For this review, take the finished solid that the model builds, in its own axes (mm). Round coordinates to 2 decimals unless told otherwise and drop trailing zeros. Order: outer loops, then holes, each group sorted by start corner. A loop starts at its lowest first (then second) coordinate and runs counter-clockwise, first axis right, second up. Notation, with made-up numbers: (-20, 31.25) - (35, 31.25) arc R15 ccw to (35, 56.25) - close; hole circle Ø3 at (0.5, 62). An arc over 180 degrees is marked (long way). Write each question's results on one line, items separated by ' | '. Start each with the question number.
(1) Take a section at C-C, the plane x = -2. Give the boundary of the cut face in (y, z).
(2) Take a section at D-D, the plane x = -51. Give the boundary of the cut face in (y, z).
(3) Take a section at A-A, the plane z = -15. Give the boundary of the cut face in (x, y), plus the area to 3 significant figures.
(4) For L1, parallel to Z at x = -38, y = 0.25; L2, parallel to Z at x = 28, y = 2.1; L3, parallel to Z at x = 12, y = 0.9, list the stretches that pass through material, from the lowest coordinate up. Write a range as from..to.
(5) Take a section at B-B, the plane y = 1.2. Give the boundary of the cut face in (x, z), plus the area to 3 significant figures.
(6) Insertion check: pin 1 Ø3 at (x, z) = (21.5, -17.5) entering from -Y. The pin has a flat end and moves straight along its axis. Give the tip position at first contact, or say it passes through.
```python
from build123d import *

# Parameters (mm, degrees)
SKETCH1_W           = 165
SKETCH1_H           = 60
BOSS_EXTRUDE1_DEPTH = 5


with BuildPart() as part:
    # Sketch1 → Boss-Extrude1 (new body)
    with BuildSketch(Plane(origin=(0, 0, 0), x_dir=(1, 0, 0), z_dir=(0, 1, 0))):
        Rectangle(SKETCH1_W, SKETCH1_H)
        Polygon((-72.5, 16.774193548), (-20.5, 0), (-72.5, -16.774193548), align=None, mode=Mode.SUBTRACT)
        Polygon((-41.5, 19.999999898), (0, 6.612903124), (41.5, 19.999999898), align=None, mode=Mode.SUBTRACT)
        Polygon((72.5, 16.774193548), (20.5, 0), (72.5, -16.774193548), align=None, mode=Mode.SUBTRACT)
        Polygon((0, -6.612903124), (41.5, -19.999999898), (-41.5, -19.999999898), align=None, mode=Mode.SUBTRACT)
    extrude(amount=BOSS_EXTRUDE1_DEPTH)


solid = part.part
```
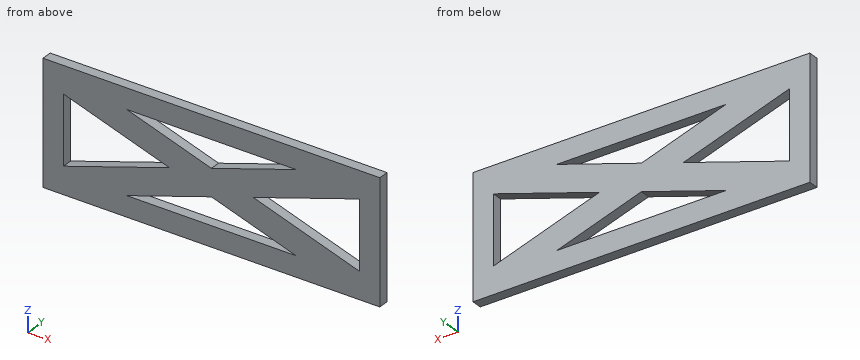
Results below:
1) outline: (0, -30) - (5, -30) - (5, -20) - (0, -20) - close; (0, -7.26) - (5, -7.26) - (5, 7.26) - (0, 7.26) - close; (0, 20) - (5, 20) - (5, 30) - (0, 30) - close
2) outline: (0, -30) - (5, -30) - (5, -9.84) - (0, -9.84) - close; (0, 9.84) - (5, 9.84) - (5, 30) - (0, 30) - close
3) outline: (-82.5, 0) - (-72.5, 0) - (-72.5, 5) - (-82.5, 5) - close; (-67, 0) - (-26, 0) - (-26, 5) - (-67, 5) - close; (26, 0) - (67, 0) - (67, 5) - (26, 5) - close; (72.5, 0) - (82.5, 0) - (82.5, 5) - (72.5, 5) - close | area: 510 mm^2
4) L1: z = -30..-20, -18.87..-5.65, 5.65..18.87, 20..30 | L2: z = -30..-20, -15.65..-2.42, 2.42..15.65, 20..30 | L3: z = -30..-20, -10.48..10.48, 20..30
5) outline: (-82.5, -30) - (82.5, -30) - (82.5, 30) - (-82.5, 30) - close; hole (-72.5, -16.77) - (-20.5, 0) - (-72.5, 16.77) - close; hole (-41.5, -20) - (41.5, -20) - (0, -6.61) - close; hole (-41.5, 20) - (0, 6.61) - (41.5, 20) - close; hole (20.5, 0) - (72.5, -16.77) - (72.5, 16.77) - close | area: 7,040 mm^2
6) pin 1: passes through
